Part model, mm, in its own coordinate system. Face numbers are marked on the shaded views. A direction names the side the tool comes from. Give positions to 0.01 mm unless a question says otherwise; leave off trailing zeros. Order: outer loops, then holes, each group sorted by start corner. A loop starts at its lowest first (then second) coordinate and runs counter-clockwise, first axis right, second up. Notation, with made-up numbers: M -20.75,18.5 L 31.25,18.5 A20 cw 31.25,27.5 Z; hole C 45,77.5 d3. An arc over 180 degrees is marked long. Return JSON: item names as keys, results as strings.
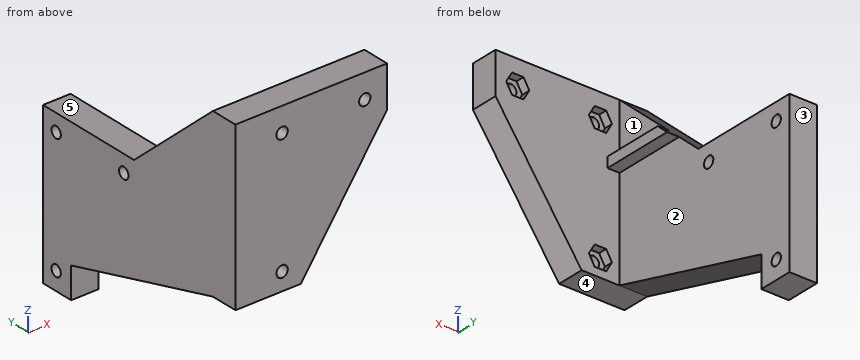
from build123d import *

# Parameters (mm, degrees)
SKETCH1_R           = 1.65
BOSS_EXTRUDE1_DEPTH = 8
SKETCH3_R           = 1.65
BOSS_EXTRUDE2_DEPTH = 8
CUT_EXTRUDE1_DEPTH  = 2.5
BOSS_EXTRUDE3_DEPTH = 3.5


with BuildPart() as part:
    # Sketch1 → Boss-Extrude1 (new body)
    with BuildSketch(Plane(origin=(0, 0, 0), x_dir=(1, 0, 0), z_dir=(0, 1, 0))):
        Polygon((-30.201635745, 21.458760302), (-19.201635745, 21.458760302), (5.798364255, -14.541239698), (5.798364255, -26.541239698), (-30.201635745, -26.541239698), align=None)
        with Locations(Location((-24.651635745, 16.308760302, 0), (0, 0, 270))):
            Circle(SKETCH1_R, mode=Mode.SUBTRACT)
        with Locations(Location((-24.651635745, -19.491239698, 0), (0, 0, 270))):
            Circle(SKETCH1_R, mode=Mode.SUBTRACT)
        with Locations(Location((-0.651635745, -19.491239698, 0), (0, 0, 270))):
            Circle(SKETCH1_R, mode=Mode.SUBTRACT)
    extrude(amount=BOSS_EXTRUDE1_DEPTH)

    # Sketch3 → Boss-Extrude2 (add)
    with BuildSketch(Plane.ZY.offset(30.201635745)):
        Polygon((-44.558757353, 58.334529743), (-35.558757353, 58.334529743), (-21.458760302, 8), (-21.458760302, 0), (26.541239698, 0), (26.541239698, 8), (1.541239698, 36), (1.541239698, 68.334529743), (-44.558757353, 68.334529743), align=None)
        with Locations((-3.458760302, 39.65)):
            Circle(SKETCH3_R, mode=Mode.SUBTRACT)
        with Locations((-3.458760302, 63.65)):
            Circle(SKETCH3_R, mode=Mode.SUBTRACT)
        with Locations((-39.258757353, 63.664529743)):
            Circle(SKETCH3_R, mode=Mode.SUBTRACT)
    extrude(amount=BOSS_EXTRUDE2_DEPTH)

    # Sketch4 → Cut-Extrude1 (cut)
    with BuildSketch(Plane(origin=(0, 8, 0), x_dir=(1, 0, 0), z_dir=(0, 1, 0))):
        Polygon((-26.326635745, 13.407575199), (-22.976635745, 13.407575199), (-21.301635745, 16.308760302), (-22.976635745, 19.209945405), (-26.326635745, 19.209945405), (-28.001635745, 16.308760302), align=None)
        Polygon((-22.976635745, -16.590054595), (-26.326635745, -16.590054595), (-28.001635745, -19.491239698), (-26.326635745, -22.392424801), (-22.976635745, -22.392424801), (-21.301635745, -19.491239698), align=None)
        Polygon((1.023364255, -16.590054595), (-2.326635745, -16.590054595), (-4.001635745, -19.491239698), (-2.326635745, -22.392424801), (1.023364255, -22.392424801), (2.698364255, -19.491239698), align=None)
    extrude(amount=-CUT_EXTRUDE1_DEPTH, mode=Mode.SUBTRACT)

    # Sketch5 → Boss-Extrude3 (add)
    with BuildSketch(Plane(origin=(-30.201635745, 0, 0), x_dir=(0, 0, -1), z_dir=(1, 0, 0))):
        Polygon((-10.641239698, 8), (-7.641239698, 8), (-7.641239698, 29.168), (-10.641239698, 25.808), align=None)
    extrude(amount=BOSS_EXTRUDE3_DEPTH)


solid = part.part
Q1. Probe line 1 along Y through (x, z) = (-31.5, -41); line 2 along Y through (x, z) = (-25.5, -9); line 3 along X through (y, z) = (61, -10). List the from-to ranges inside material, lowest first.
Established:
{"line 1": "y = 58.33 to 68.33", "line 2": "y = 0 to 8", "line 3": "x = -38.2 to -30.2"}
Q2. Band-saw the part on D-D (x = -11). Give the cut face in (y, z).
Established:
{"outline": "M 0,-9.65 L 8,-9.65 L 8,26.54 L 0,26.54 Z"}
Q3. 3-axis set-ups, long thin cutter, end or side, ignore diameter. For the marked faces 1, 2, 3, 4 and 5: which of +Z, -Z, +X, -X, +Y, -Y reach the whole face in a straight line?
Established:
{"face 1": "+Z, +X, +Y", "face 2": "-Z, +X, +Y", "face 3": "+Z, -Z, +X, -X, +Y", "face 4": "-Z, +X, -X, -Y", "face 5": "+Z, +X, -X, +Y"}
Q4. Band-saw the part on A-A (y = 39.65). Give the cut face in (x, z).
Established:
{"outline": "M -38.2,-30.32 L -30.2,-30.32 L -30.2,-5.11 L -38.2,-5.11 Z; M -38.2,-1.81 L -30.2,-1.81 L -30.2,1.54 L -38.2,1.54 Z"}
Q5. Pin check, flat tips, straight feed: pin 1 (4.5 mm diameter, centred on x = -24.65, z = -16.31, fed in from +Y); pin 2 (1 mm diameter, centred on x = -29, y = 18, fed in from -Z); pin 3 (2.5 mm diameter, centred on x = -35.5, y = 48, fed in from +Z); pin 4 (6 mm diameter, centred on x = -25.5, y = 50, fed in from -Z). Stop position of each tip, or through.
Established:
{"pin 1": "stops at y = 5.5", "pin 2": "stops at z = 7.64", "pin 3": "stops at z = 1.54", "pin 4": "passes through"}
Q6. Band-saw the part on B-B (x = -32.5). Give the cut face in (y, z), then the cut area to 3 significant figures.
Established:
{"outline": "M 0,-21.46 L 8,-21.46 L 58.33,-35.56 L 58.33,-44.56 L 68.33,-44.56 L 68.33,1.54 L 36,1.54 L 8,26.54 L 0,26.54 Z; hole C 39.65,-3.46 d3.3; hole C 63.65,-3.46 d3.3; hole C 63.66,-39.26 d3.3", "area": "2,680 mm²"}
Q7. Band-saw the part on C-C (z = 5). Give the cut face in (x, y), then the cut area to 3 significant figures.
Established:
{"outline": "M -38.2,0 L -0.83,0 L -0.83,8 L -30.2,8 L -30.2,32.13 L -38.2,32.13 Z", "area": "492 mm²"}
